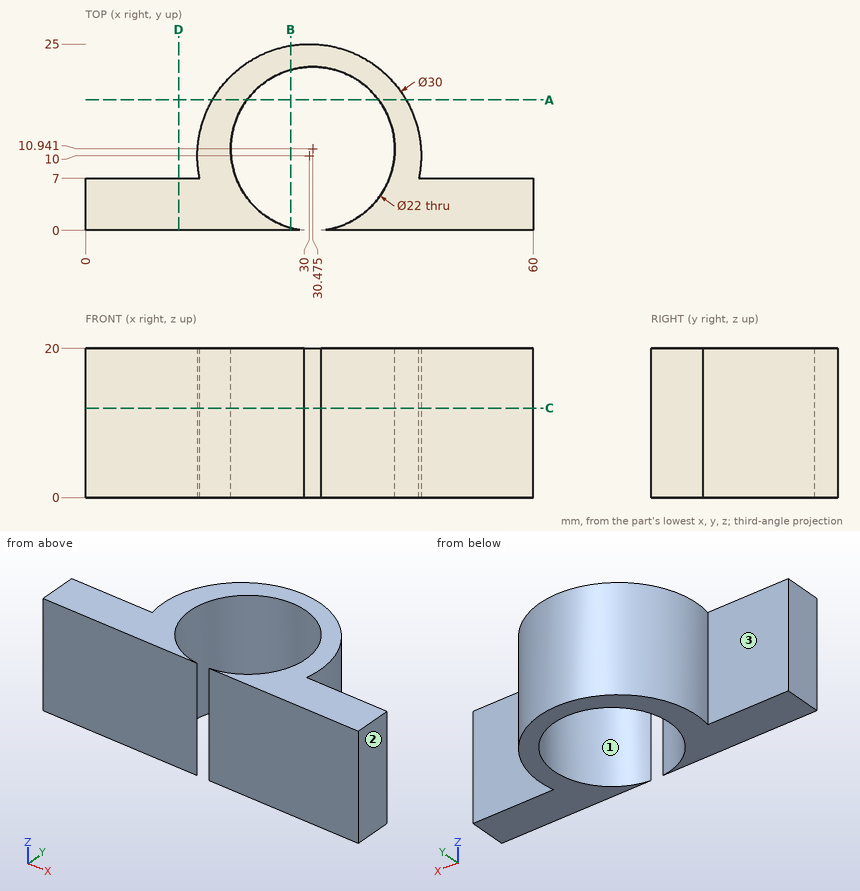
Design review of the part shown in the three views and the two pictorial views. Dimensions are in mm from the part's minimum x, y and z. Round coordinates to 2 decimals unless told otherwise and drop trailing zeros. Loops run counter-clockwise (first coordinate to the right, second up) from the corner with the lowest first, then second, coordinate; pieces in that order, holes last. Notation, with made-up numbers: M -8,39 L 33,39 A25 ccw 33,52 Z; hole C 43.25,-17.5 d6. An arc over 180 degrees is marked long. Answer as a JSON object with one key per item and string values.
Item 1: We need section C-C on z = 12. Give the boundary of the cut face in (x, y) (1 decimal), and give its area (3 significant figures).
Answer sheet:
{"outline": "M 0,0 L 29.3,0 A11 cw long 31.6,0 L 60,0 L 60,7 L 44.7,7 A15 ccw long 15.3,7 L 0,7 Z", "area": "483 mm^2"}
Item 2: We need section D-D on x = 12.5. Give the boundary of the cut face in (y, z), and give its area (3 significant figures).
Answer sheet:
{"outline": "M 0,0 L 7,0 L 7,20 L 0,20 Z", "area": "140 mm^2"}
Item 3: Wall thickness on L1, parallel to Y at x = 3.5, z = 9.5; L2, parallel to X at y = 10, z = 9 (1 decimal); L3, parallel to X at y = 2.5, z = 4.5: over which ranges is each line inside the solid? List them lowest first. Write a range as from..to.
Answer sheet:
{"L1": "y = 0..7", "L2": "x = 15..19.5, 41.4..45", "L3": "x = 0..23.42, 37.53..60"}
Item 4: We need section A-A on y = 17.5. Give the boundary of the cut face in (x, z) (1 decimal).
Answer sheet:
{"outline": "M 17,0 L 21.6,0 L 21.6,20 L 17,20 Z; M 39.3,0 L 43,0 L 43,20 L 39.3,20 Z"}
Item 5: Clearance check with flat-ended pins moving along their axes: P1, Ø4.5, axis at x = 6.5, z = 9.5, coming from the +Y side; P2, Ø12, axis at x = 13, y = 19.5, coming from the +Z side; P3, Ø3, axis at y = 14, z = 3, coming from the +X side. State where each tip first meets the part, or that it passes through.
Answer sheet:
{"P1": "stops at y = 7", "P2": "stops at z = 20", "P3": "stops at x = 44.79"}
Item 6: The part is to be moulded in two halves that separate along X. For the marked faces 1, 2 and 3, say which applies: pulls with the +X half, pulls with the -X half, needs draft (parallel to the pull), parting line crosses it, or undercut.
Answer sheet:
{"face 1": "undercut", "face 2": "pulls with the +X half", "face 3": "needs draft"}
Item 7: We need section B-B on x = 27.5. Give the boundary of the cut face in (y, z).
Answer sheet:
{"outline": "M 0,0 L 0.35,0 L 0.35,20 L 0,20 Z; M 21.53,0 L 24.79,0 L 24.79,20 L 21.53,20 Z"}
